CAD build for the part. Positions are in the model's coordinates, mm. Coordinates: 2 decimals unless noted, no trailing zeros. Loops run counter-clockwise (first coordinate to the right, second up) from the corner with the lowest first, then second, coordinate; pieces in that order, holes last. Notation, with made-up numbers: (30.5, 56) -> (84.5, 56) arc R21 cw to (84.5, 70) -> close; hole circle Ø2 at (40, 69). An arc over 180 degrees is marked (long way). Answer as CSV lines item,"result". Start each with the question number.
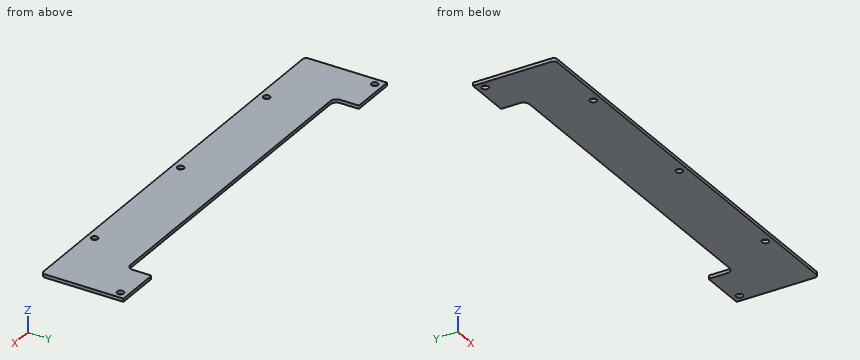
from build123d import *

# Parameters (mm, degrees)
F0_W     = 224.7782652
F0_H     = 43.0059846
F0_R     = 1.7272
F1_DEPTH = 1.70942
F2_R     = 1.98374
F3_W     = 176.9053931614
F3_H     = 12.9915969446
F4_DEPTH = 1.70942
F5_R     = 3.175
F6_R     = 0.762


with BuildPart() as f1:
    # F0 (on Top) → F1 (new body)
    with BuildSketch(Plane.XY):
        with Locations((112.3891326, -21.5029923)):
            Rectangle(F0_W, F0_H)
        with Locations((39.0372346, -39.0372346)):
            Circle(F0_R, mode=Mode.SUBTRACT)
        with Locations((112.3891326, -39.0372346)):
            Circle(F0_R, mode=Mode.SUBTRACT)
        with Locations((185.7410306, -39.0372346)):
            Circle(F0_R, mode=Mode.SUBTRACT)
        with Locations((3.96875, -3.96875)):
            Circle(F0_R, mode=Mode.SUBTRACT)
        with Locations((220.8095152, -3.96875)):
            Circle(F0_R, mode=Mode.SUBTRACT)
    extrude(amount=F1_DEPTH)

    # F2
    f2_edges = [f1.edges().sort_by_distance(p)[0] for p in [
        (0, -43.005985, 0.85471),
        (224.778265, -43.005985, 0.85471),
    ]]
    fillet(f2_edges, radius=F2_R)

    # F3 (on face) → F4 (cut, through all)
    with BuildSketch(Plane.XY.offset(1.70942)):
        with Locations((112.3891326, -6.4957984723)):
            Rectangle(F3_W, F3_H)
    extrude(amount=-F4_DEPTH, mode=Mode.SUBTRACT)

    # F5
    f5_edges = [f1.edges().sort_by_distance(p)[0] for p in [
        (200.841829, -12.991597, 0.85471),
        (23.936436, -12.991597, 0.85471),
    ]]
    fillet(f5_edges, radius=F5_R)

    # F6
    f6_edges = [f1.edges().sort_by_distance(p)[0] for p in [
        (23.936436, 0, 0.85471),
        (200.841829, 0, 0.85471),
    ]]
    fillet(f6_edges, radius=F6_R)


solid = f1.part
Item 1: Saw through at A-A (z = 0.55). Write the cut outline in (x, y) (3 decimals).
Item 2: Saw through at B-B (x = 62.5). Write the cut outline in (y, z), plus the area to 3 significant figures.
Item 3: Flat gauge pins, fed straight in: pin 1 Ø5 at (x, y) = (111.5, -8) entering from +Z; pin 2 Ø3 at (x, y) = (132.5, -20.5) entering from -Z; pin 3 Ø0.5 at (x, z) = (121.5, 0.5) entering from +Y. Where does each tip first touch, or does it go through?
Item 4: Wall check: probe 1 along X at (y, z) = (-6.5, 0.4); probe 2 along X at (y, z) = (-39.5, 1.25); probe 3 along Y at (x, z) = (103, 0.65). Give the ranges that are in metal, low to high.
Geometry check:
1,outline,"(0, -41.022) arc R1.984 ccw to (1.984, -43.006) -> (222.795, -43.006) arc R1.984 ccw to (224.778, -41.022) -> (224.778, 0) -> (201.604, 0) arc R0.762 ccw to (200.842, -0.762) -> (200.842, -9.817) arc R3.175 cw to (197.667, -12.992) -> (27.111, -12.992) arc R3.175 cw to (23.936, -9.817) -> (23.936, -0.762) arc R0.762 ccw to (23.174, 0) -> (0, 0) -> close; hole circle Ø3.454 at (3.969, -3.969); hole circle Ø3.454 at (39.037, -39.037); hole circle Ø3.454 at (112.389, -39.037); hole circle Ø3.454 at (185.741, -39.037); hole circle Ø3.454 at (220.81, -3.969)"
2,outline,"(-43.01, 0) -> (-12.99, 0) -> (-12.99, 1.71) -> (-43.01, 1.71) -> close"
2,area,"51.3 mm2"
3,pin 1,"through"
3,pin 2,"z = 0"
3,pin 3,"y = -12.99"
4,probe 1,"0 to 23.94, 200.84 to 224.78"
4,probe 2,"0 to 37.37, 40.7 to 110.73, 114.05 to 184.08, 187.41 to 224.78"
4,probe 3,"-43.01 to -12.99"
